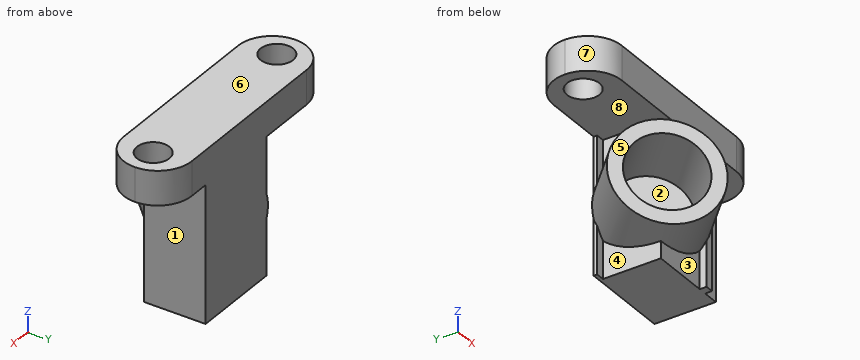
```python
from build123d import *

# Parameters (mm, degrees)
SKETCH1_W           = 35
SKETCH1_H           = 10
SKETCH1_R           = 2.38125
BOSS_EXTRUDE1_DEPTH = 5
BOSS_EXTRUDE2_DEPTH = 20
SKETCH3_R           = 5.5
CUT_EXTRUDE1_DEPTH  = 6
BOSS_EXTRUDE3_START = 10
SKETCH4_R           = 7.5
SKETCH4_R_2         = 5.5
BOSS_EXTRUDE3_DEPTH = 10
FILLET1_R           = 5
BOSS_EXTRUDE4_START = -20
SKETCH5_W           = 1.25
SKETCH5_H           = 0.514718626
BOSS_EXTRUDE4_DEPTH = 20
SKETCH6_W           = 6.624212501
SKETCH6_H           = 0.612418682
CUT_EXTRUDE2_DEPTH  = 33.839440066
BOSS_EXTRUDE5_START = -20
SKETCH7_W           = 1.18849251
SKETCH7_H           = 1
BOSS_EXTRUDE5_DEPTH = 20


with BuildPart() as part:
    # Sketch1 → Boss-Extrude1 (new body)
    with BuildSketch(Plane.XY):
        Rectangle(SKETCH1_W, SKETCH1_H)
        with Locations((13.5, 0)):
            Circle(SKETCH1_R, mode=Mode.SUBTRACT)
        with Locations(Location((-13.5, 0, 0), (0, 0, 180))):
            Circle(SKETCH1_R, mode=Mode.SUBTRACT)
    extrude(amount=BOSS_EXTRUDE1_DEPTH)

    # Sketch2 → Boss-Extrude2 (add)
    with BuildSketch(Plane(origin=(0, 0, 0), x_dir=(-1, 0, 0), z_dir=(0, 0, -1))):
        Polygon((-9.5, -4), (2.5, -4), (2.5, 4), (2.5, 5), (-9.5, 5), (-9.5, 4), align=None)
    extrude(amount=BOSS_EXTRUDE2_DEPTH)

    # Sketch3 → Cut-Extrude1 (cut)
    with BuildSketch(Plane(origin=(-3.25, -3.25, 0), x_dir=(0, 0, 1), z_dir=(-0.7071067811865488, -0.7071067811865464, 0))):
        with Locations(Location((-10, -1.060660172, 0), (0, 0, 270))):
            Circle(SKETCH3_R)
    extrude(amount=-CUT_EXTRUDE1_DEPTH, mode=Mode.SUBTRACT)

    # Sketch4 → Boss-Extrude3 (add)
    with BuildSketch(Plane(origin=(0.992640687, 0.992640687, 0), x_dir=(0, 0, 1), z_dir=(-0.7071067811865488, -0.7071067811865462, 0)).offset(BOSS_EXTRUDE3_START)):
        with Locations(Location((-10, -1.060660172, 0), (0, 0, 53.130102354))):
            Circle(SKETCH4_R)
        with Locations(Location((-10, -1.060660172, 0), (0, 0, 270))):
            Circle(SKETCH4_R_2, mode=Mode.SUBTRACT)
    extrude(amount=-BOSS_EXTRUDE3_DEPTH)

    # Fillet1
    fillet1_edges = [part.edges().sort_by_distance(p)[0] for p in [
        (17.5, 5, 2.5),
        (17.5, -5, 2.5),
        (-17.5, -5, 2.5),
        (-17.5, 5, 2.5),
    ]]
    fillet(fillet1_edges, radius=FILLET1_R - 0.0001)  # a hair under: the kernel refuses the full size

    # Sketch5 → Boss-Extrude4 (add)
    with BuildSketch(Plane(origin=(0, 0, -20), x_dir=(-1, 0, 0), z_dir=(0, 0, -1)).offset(BOSS_EXTRUDE4_START)):
        with Locations((3.125, 4.742640687)):
            Rectangle(SKETCH5_W, SKETCH5_H)
    extrude(amount=BOSS_EXTRUDE4_DEPTH)

    # Sketch6 → Cut-Extrude2 (cut, through all)
    with BuildSketch(Plane(origin=(0, 0, -20), x_dir=(-1, 0, 0), z_dir=(0, 0, -1))):
        with Locations((6.326824877, 5.306209341)):
            Rectangle(SKETCH6_W, SKETCH6_H)
    extrude(amount=-CUT_EXTRUDE2_DEPTH, mode=Mode.SUBTRACT)

    # Sketch7 → Boss-Extrude5 (add)
    with BuildSketch(Plane(origin=(0, 0, -20), x_dir=(-1, 0, 0), z_dir=(0, 0, -1)).offset(BOSS_EXTRUDE5_START)):
        with Locations((-6.579527629, -4.5)):
            Rectangle(SKETCH7_W, SKETCH7_H)
    extrude(amount=BOSS_EXTRUDE5_DEPTH)


solid = part.part
```
Source: CAD feature listing. Evaluate the final solid. Frame: model axes, mm. Face numbers are marked on the shaded views. A direction names the side the tool comes from. Round coordinates to 2 decimals unless told otherwise and drop trailing zeros. Loops run counter-clockwise (first coordinate to the right, second up) from the corner with the lowest first, then second, coordinate; pieces in that order, holes last.
(1) Section query C-C (z = -10.5). Output: boundary loops of the cut face in (x, y).
From the geometry:
outline: (-10.62, -1.54) - (-9.2, -2.96) - (-2.13, 4.12) - (5.62, -3.63) - (-1.46, -10.7) - (-0.04, -12.12) - (7.03, -5.05) - (6.99, -5) - (7.17, -5) - (7.17, -4) - (9.5, -4) - (9.5, 5) - (-4.08, 5) - close
(2) Material intervals for probe 1 along Z at (x, y) = (-3, -4.5); probe 2 along Z at (x, y) = (-5, -0.25); probe 3 along X at (y, z) = (-0.25, -10.25), sorted ascending.
From the geometry:
probe 1: z = -17.5 to -15.5, -4.5 to -2.5, 0 to 5
probe 2: z = -16.06 to -13.27, -6.73 to -3.94, 0 to 5
probe 3: x = -9.35 to -6.52, 2.24 to 9.5
(3) Section query A-A (z = 2.25). Give the number of separate pieces and of enclosed holes in the cut face, and give its area (3 significant figures).
From the geometry:
separate pieces: 1
enclosed holes: 2
area: 293 mm2
(4) Contact query for flat-ended pins moving along their axis: pin 1 Ø3 at (x, y) = (13.5, 0) entering from +Z; pin 2 Ø0.6 at (x, z) = (-3, -15) entering from -Y; pin 3 Ø1.7 at (y, z) = (0.5, -2) entering from -X; pin 4 Ø3 at (y, z) = (-1.5, -16) entering from -X. Output: stop coordinate, or through.
From the geometry:
pin 1: passes through
pin 2: stops at y = -9.46
pin 3: stops at x = -2.5
pin 4: stops at x = -9.05
(5) Pull-direction query (Z, two-part tool) for the marked faces 6, 7 and 8; classes: +Z half, -Z half, draft (parallel to the pull), parting line (faces both ways), or undercut.
From the geometry:
face 6: +Z half
face 7: draft
face 8: undercut
(6) Section query B-B (x = 13.5). Output: boundary loops of the cut face in (y, z).
From the geometry:
outline: (-4.9, 0) - (-2.38, 0) - (-2.38, 5) - (-4.9, 5) - close; (2.38, 0) - (4.9, 0) - (4.9, 5) - (2.38, 5) - close
(7) Access query for the marked faces 1, 2, 3, 4 and 5. Directions: +Z, -Z, +X, -X, +Y, -Y. A direction counts if a zero-diameter tool reaches every point of the face in a straight line with its end or side. Return the directions, or none.
From the geometry:
face 1: -Z, +X, +Y, -Y
face 2: none
face 3: -Z, -Y
face 4: -Z, -X
face 5: -Z, -X, -Y
